Build history of the part. All positions in model axes, mm. A direction names the side the tool comes from. Round coordinates to 2 decimals unless told otherwise and drop trailing zeros. Write each loop counter-clockwise with the first axis right and the second up, starting at its lowest first coordinate (ties: lowest second). Pieces come first, ordered by that corner, then holes. Notation, with made-up numbers: (-35, 52) -> (1, 52) arc R19 cw to (1, 59) -> close; hole circle Ø6 at (21, 87.5). An arc over 180 degrees is marked (long way). Return JSON: item names as keys, results as strings.
from build123d import *

# Parameters (mm, degrees)
BOSS_EXTRUDE1_DEPTH = 3.9624
CUT_EXTRUDE1_DEPTH  = 0.0508


with BuildPart() as part:
    # Sketch1 → Boss-Extrude1 (new body)
    with BuildSketch(Plane(origin=(0, 0, 0), x_dir=(1, 0, 0), z_dir=(0, 1, 0))):
        Polygon((6.415804866, 0), (3.207902433, 5.55625), (-3.207902433, 5.55625), (-6.415804866, 0), (-3.207902433, -5.55625), (3.207902433, -5.55625), align=None)
    extrude(amount=BOSS_EXTRUDE1_DEPTH)

    # Sketch2 → Cut-Revolve1 (revolve, cut)
    with BuildSketch(Plane.XY):
        Polygon((5.55625, 3.9624), (6.415804866, 3.4544), (6.415804866, 3.9624), align=None)
    revolve(axis=Axis((0, 0, 0), (0, 1, 0)), mode=Mode.SUBTRACT)

    # Sketch3 → Cut-Extrude1 (cut)
    with BuildSketch(Plane(origin=(0, 3.9624, 0), x_dir=(-1, 0, 0), z_dir=(0, -1, 0))):
        with BuildLine():
            Line((0.127, 4.7625), (0.127, 2.7305))
            ThreePointArc((0.127, 2.7305), (0, 2.6035), (-0.127, 2.7305))
            Line((-0.127, 2.7305), (-0.127, 4.7625))
            ThreePointArc((-0.127, 4.7625), (0, 4.8895), (0.127, 4.7625))
        make_face()
        with BuildLine():
            Line((4.060945986, -2.491235226), (2.301182365, -1.475235226))
            ThreePointArc((2.301182365, -1.475235226), (2.254697139, -1.30175), (2.428182365, -1.255264774))
            Line((2.428182365, -1.255264774), (4.187945986, -2.271264774))
            ThreePointArc((4.187945986, -2.271264774), (4.234431212, -2.44475), (4.060945986, -2.491235226))
        make_face()
        with BuildLine():
            Line((-4.187945986, -2.271264774), (-2.428182365, -1.255264774))
            ThreePointArc((-2.428182365, -1.255264774), (-2.254697139, -1.30175), (-2.301182365, -1.475235226))
            Line((-2.301182365, -1.475235226), (-4.060945986, -2.491235226))
            ThreePointArc((-4.060945986, -2.491235226), (-4.234431212, -2.44475), (-4.187945986, -2.271264774))
        make_face()
    extrude(amount=CUT_EXTRUDE1_DEPTH, mode=Mode.SUBTRACT)

    # Bolt Length Sketch → Bolt Length (revolve)
    with BuildSketch(Plane.XY):
        Polygon((0, 0), (0, -69.85), (2.778125, -69.85), (3.175, -69.215), (3.175, 0), align=None)
    revolve(axis=Axis((0, 0, 0), (0, -1, 0)))


solid = part.part
Q1. Pin check, flat tips, straight feed: pin 1 Ø2 at (y, z) = (-34, 3) entering from -X; pin 2 Ø1 at (y, z) = (-14, 0.5) entering from +X (3 decimals); pin 3 Ø5 at (y, z) = (-45, -3.5) entering from -X. Stop position of each tip, or through.
Verdict:
{"pin 1": "stops at x = -2.47", "pin 2": "stops at x = 3.175", "pin 3": "stops at x = -3.01"}
Q2. Wall check: L1, parallel to X at y = -28, z = -0.25; L2, parallel to X at y = -55.5, z = 2.25. Give the ranges that are in metal, low to high.
Verdict:
{"L1": "x = -3.17 to 3.17", "L2": "x = -2.24 to 2.24"}
Q3. 3-axis set-ups, long thin cutter, end or side, ignore diameter. For faces 1 (the flat face through (0, 2, 5.556)), 2 (the flat face through (3, 0, -3)): which of +Z, -Z, +X, -X, +Y, -Y reach the whole face in a straight line?
Verdict:
{"face 1": "+Z, +X, -X, +Y, -Y", "face 2": "-Y"}
Q4. Saw through at A-A on y = -19.5. List the corners of the cut face in (x, z) (3 decimals).
Verdict:
{"outline": "circle Ø6.35 at (0, 0)"}
